For this review, use the dimensioned drawing (mm, ordinates from the lowest corner) and the shaded views. Coordinates: 2 decimals unless noted, no trailing zeros. Order: outer loops, then holes, each group sorted by start corner. A loop starts at its lowest first (then second) coordinate and runs counter-clockwise, first axis right, second up. Notation, with made-up numbers: M 77.5,45.5 L 87.5,45.5 A20 ccw 87.5,49.5 Z; hole C -21.5,-18 d10. An arc over 180 degrees is marked long. Answer in a Markdown table with one row per item.
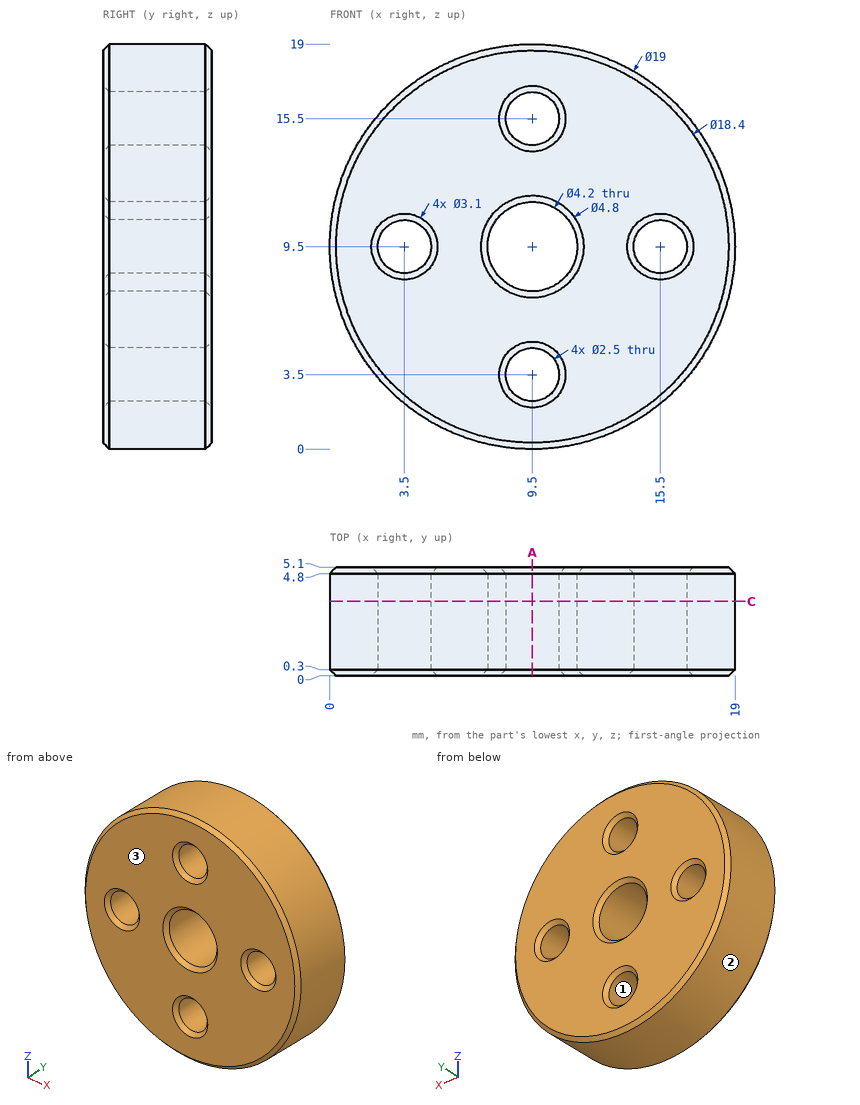
(1) Take a section at C-C (y = 3.5). Write out the cut boundary in (x, z), then the cut area to 3 significant figures.
Report:
| item | result |
|---|---|
| outline | C 9.5,9.5 d19; hole C 3.5,9.5 d2.5; hole C 9.5,9.5 d4.2; hole C 9.5,3.5 d2.5; hole C 9.5,15.5 d2.5; hole C 15.5,9.5 d2.5 |
| area | 250 mm^2 |
(2) Take a section at A-A (x = 9.5). State how many separate pieces and enclosed holes the cut face has, then the cut area to 3 significant figures.
Report:
| item | result |
|---|---|
| separate pieces | 4 |
| enclosed holes | 0 |
| area | 49.3 mm^2 |
(3) Insertion check: P1, Ø2, axis at y = 0.5, z = 2, coming from the -X side; P2, Ø2, axis at x = 3.5, z = 9.5, coming from the -Y side; P3, Ø1.5, axis at x = 10.5, y = 3, coming from the +Z side; P4, Ø3, axis at x = 9.5, z = 3.5, coming from the -Y side. Each pin has a flat end and moves straight along its axis. Give the tip position at first contact, or say it passes through.
Report:
| item | result |
|---|---|
| P1 | x = 2.57 |
| P2 | through |
| P3 | z = 19 |
| P4 | y = 0.05 |
(4) The part is to be moulded in two halves that separate along X. For the marked faces 1, 2 and 3, say which applies: +X half, -X half, draft (parallel to the pull), parting line (faces both ways), or undercut.
Report:
| item | result |
|---|---|
| face 1 | undercut |
| face 2 | parting line |
| face 3 | draft |
(5) To check wall thickness, follow line 1 (X direction, y = 1.8, z = 9.5); line 2 (Z direction, x = 14.5, y = 4.15). State the ranges of each line that lie inside material, in increasing order. Write a range as [from, to].
Report:
| item | result |
|---|---|
| line 1 | [0, 2.25], [4.75, 7.4], [11.6, 14.25], [16.75, 19] |
| line 2 | [1.42, 8.75], [10.25, 17.58] |
